The listing builds one solid part. Answer for the finished solid, in the listing's coordinates (mm). A direction names the side the tool comes from. Round coordinates to 2 decimals unless told otherwise and drop trailing zeros. Write each loop counter-clockwise with the first axis right and the second up, starting at its lowest first coordinate (ties: lowest second). Pieces come first, ordered by that corner, then holes. Notation, with made-up numbers: M 9.25,89 L 19.25,89 A26 ccw 19.25,122 Z; hole C -8.75,21.25 d5. An arc over 180 degrees is marked long. Write each question's results on one line, items separated by ' | '.
from build123d import *

# Parameters (mm, degrees)
BOSS_EXTRUDE1_DEPTH = 6.35
CUT_EXTRUDE1_REACH  = 45.068
SKETCH2_R           = 3.175
CUT_EXTRUDE2_START  = -6.35
SKETCH4_R           = 0.635
CUT_EXTRUDE2_DEPTH  = 6.35


with BuildPart() as part:
    # Sketch1 → Boss-Extrude1 (new body)
    with BuildSketch(Plane(origin=(0, 0, 0), x_dir=(1, 0, 0), z_dir=(0, 1, 0))):
        Polygon((-19.05, 12.7), (-19.05, 19.05), (-6.35, 19.05), (-6.35, 12.7), (6.35, 12.7), (6.35, 19.05), (19.05, 19.05), (19.05, 12.7), (38.1, 12.7), (38.1, -12.7), (19.05, -12.7), (19.05, -19.05), (6.35, -19.05), (6.35, -12.7), (-6.35, -12.7), (-6.35, -19.05), (-19.05, -19.05), (-19.05, -12.7), (-38.1, -12.7), (-38.1, 12.7), align=None)
    extrude(amount=BOSS_EXTRUDE1_DEPTH)

    # Sketch2 → Cut-Extrude1 (cut, up to next)
    with BuildSketch(Plane(origin=(0, 6.35, 0), x_dir=(1, 0, 0), z_dir=(0, 1, 0)), mode=Mode.PRIVATE) as cut_extrude1_sk1:
        with Locations(Location((-12.7, 0, 0), (0, 0, 270))):
            Circle(SKETCH2_R)
    cut_extrude1_tool1 = extrude(cut_extrude1_sk1.sketch, amount=-CUT_EXTRUDE1_REACH, mode=Mode.PRIVATE) & part.part
    # Sketch2 → Cut-Extrude1 (cut, up to next)
    with BuildSketch(Plane(origin=(0, 6.35, 0), x_dir=(1, 0, 0), z_dir=(0, 1, 0)), mode=Mode.PRIVATE) as cut_extrude1_sk2:
        with Locations(Location((12.7, 0, 0), (0, 0, 270))):
            Circle(SKETCH2_R)
    cut_extrude1_tool2 = extrude(cut_extrude1_sk2.sketch, amount=-CUT_EXTRUDE1_REACH, mode=Mode.PRIVATE) & part.part
    add(cut_extrude1_tool1.solids().sort_by_distance((-12.7, 6.35, 0))[0], mode=Mode.SUBTRACT)
    add(cut_extrude1_tool2.solids().sort_by_distance((12.7, 6.35, 0))[0], mode=Mode.SUBTRACT)

    # Sketch4 → Cut-Extrude2 (cut)
    with BuildSketch(Plane(origin=(0, 6.35, 0), x_dir=(1, 0, 0), z_dir=(0, 1, 0)).offset(CUT_EXTRUDE2_START)):
        with Locations((-19.05, 12.7)):
            Circle(SKETCH4_R)
    cut_extrude2 = extrude(amount=CUT_EXTRUDE2_DEPTH, mode=Mode.SUBTRACT)

    # Sketch-Pattern1: Cut-Extrude2 at 7 more places
    with Locations((12.7, 0, 0), (25.4, 0, 0), (38.1, 0, 0), (38.1, 0, 25.4), (25.4, 0, 25.4), (12.7, 0, 25.4), (0, 0, 25.4)):
        add(cut_extrude2, mode=Mode.SUBTRACT)


solid = part.part
1) Each of these flat-tipped pins is pushed along its axis until it touches: pin 1 (3 mm diameter, centred on x = 23, y = 1, fed in from -Z); pin 2 (0.8 mm diameter, centred on x = 19.05, z = -12.7, fed in from +Y); pin 3 (3 mm diameter, centred on x = 1.5, y = 4, fed in from +Z); pin 4 (1.7 mm diameter, centred on y = 2.5, z = -17.5, fed in from -X). Where does it stop, or does it pass through?
Return value:
pin 1: z = -12.7 | pin 2: through | pin 3: z = 12.7 | pin 4: x = -19.05
2) Section B-B (x = -12.7) is taken. Determine the outline of the cut face in (y, z) (3 decimals), then the cut area to 3 significant figures.
Return value:
outline: M 0,-19.05 L 6.35,-19.05 L 6.35,-3.175 L 0,-3.175 Z; M 0,3.175 L 6.35,3.175 L 6.35,19.05 L 0,19.05 Z | area: 202 mm²
3) A tool of negligible diameter and unlimited length cuts with its end or side. For faces 1 (the face through (-6.35, 3, 16)), 2 (the face through (-19.05, 3, 16)), 3 (the face through (29, 3, 12.7)), 4 (the face through (0, 3, -12.7)), from which of +Z, -Z, +X, -X, +Y, -Y can it reach the whole face along a straight path? Write none if from no direction.
Return value:
face 1: +Z, +Y, -Y | face 2: +Z, -X, +Y, -Y | face 3: +Z, +X, +Y, -Y | face 4: -Z, +Y, -Y
4) The mould has two halves that part along X. Classify faces 5 (the face through (-38.1, 3, 0)), 6 (the face through (6.35, 3, -16)), 7 (the face through (13, 3, 19.05)): +X half, -X half, draft (parallel to the pull), parting line (faces both ways), or undercut.
Return value:
face 5: -X half | face 6: undercut | face 7: draft
5) Section C-C (z = -16) is taken. Determine the outline of the cut face in (x, y).
Return value:
outline: M -19.05,0 L -6.35,0 L -6.35,6.35 L -19.05,6.35 Z; M 6.35,0 L 19.05,0 L 19.05,6.35 L 6.35,6.35 Z
6) Section A-A (z = 0) is taken. Determine the outline of the cut face in (x, y) (3 decimals), then the cut area to 3 significant figures.
Return value:
outline: M -38.1,0 L -15.875,0 L -15.875,6.35 L -38.1,6.35 Z; M -9.525,0 L 9.525,0 L 9.525,6.35 L -9.525,6.35 Z; M 15.875,0 L 38.1,0 L 38.1,6.35 L 15.875,6.35 Z | area: 403 mm²
7) Section D-D (y = 4.5) is taken. State how many separate pieces and enclosed holes the cut face has, then the cut area to 3 significant figures.
Return value:
separate pieces: 1 | enclosed holes: 2 | area: 2,190 mm²
8) Find the intervals of material crossed by line 1 (X direction, y = 3.75, z = 0) (3 decimals); line 2 (X direction, y = 3.25, z = 17.5); line 3 (Z direction, x = 15, y = 4.5), in increasing order.
Return value:
line 1: -38.1 to -15.875, -9.525 to 9.525, 15.875 to 38.1 | line 2: -19.05 to -6.35, 6.35 to 19.05 | line 3: -19.05 to -2.19, 2.19 to 19.05
